```python
from build123d import *
from OCP.BRepFilletAPI import BRepFilletAPI_MakeChamfer

# Parameters (mm, degrees)
SKETCH2_W           = 18
SKETCH2_H           = 20
BOSS_EXTRUDE1_DEPTH = 22
SKETCH3_W           = 18
SKETCH3_H           = 20
BOSS_EXTRUDE2_DEPTH = 8
BOSS_EXTRUDE2_DRAFT = -25
SKETCH4_R           = 1.6
CUT_EXTRUDE1_DEPTH  = 18
CHAMFER1_SIZE       = 0.4
CHAMFER1_SIZE2      = 0.300994928


with BuildPart() as part:
    # Sketch2 → Boss-Extrude1 (new body)
    with BuildSketch(Plane.XY):
        Rectangle(SKETCH2_W, SKETCH2_H)
    extrude(amount=BOSS_EXTRUDE1_DEPTH)


with BuildPart() as boss_extrude2_tool:
    # Sketch3 → Boss-Extrude2 (with draft: the straight prism first)
    with BuildSketch(Plane(origin=(0, 0, 0), x_dir=(-1, 0, 0), z_dir=(0, 0, -1))):
        Rectangle(SKETCH3_W, SKETCH3_H)
    extrude(amount=BOSS_EXTRUDE2_DEPTH)
    # Boss-Extrude2: the draft: its side faces are tilted about the plane it starts from
    boss_extrude2_sides = [boss_extrude2_tool.faces().sort_by_distance(p)[0] for p in [
        (9, 0, -4),
        (0, -10, -4),
        (-9, 0, -4),
        (0, 10, -4),
    ]]
    draft(boss_extrude2_sides, Plane(origin=(0, 0, 0), x_dir=(-1, 0, 0), z_dir=(0, 0, -1)), BOSS_EXTRUDE2_DRAFT)


with BuildPart() as part_1:
    add(part.part)

    # Boss-Extrude2: add boss_extrude2_tool
    add(boss_extrude2_tool.part)

    # Sketch4 → Cut-Extrude1 (cut)
    with BuildSketch(Plane(origin=(9, 0, 0), x_dir=(0, 0, -1), z_dir=(1, 0, 0))):
        with Locations((-17, 5)):
            Circle(SKETCH4_R)
        with Locations((-9, 5)):
            Circle(SKETCH4_R)
        with Locations((-17, -5)):
            Circle(SKETCH4_R)
        with Locations((-9, -5)):
            Circle(SKETCH4_R)
    extrude(amount=-CUT_EXTRUDE1_DEPTH, mode=Mode.SUBTRACT)

    # Chamfer1: one chamfer whose edges measure the first distance from different faces: ONE call of the kernel's chamfer builder (chamfer() names one face for all edges)
    chamfer1_edges_1 = [part_1.edges().sort_by_distance(p)[0] for p in [
        (0, 13.730461265, -8),
    ]]
    chamfer1_side_1 = [part_1.faces().sort_by_distance(p)[0] for p in [
        (0, 11.971965146, -4.228892903),
    ]]
    chamfer1_edges_2 = [part_1.edges().sort_by_distance(p)[0] for p in [
        (12.730461265, 0, -8),
    ]]
    chamfer1_side_2 = [part_1.faces().sort_by_distance(p)[0] for p in [
        (10.962969576, 0, -4.20960184),
    ]]
    chamfer1_edges_3 = [part_1.edges().sort_by_distance(p)[0] for p in [
        (0, -13.730461265, -8),
    ]]
    chamfer1_side_3 = [part_1.faces().sort_by_distance(p)[0] for p in [
        (0, -11.971965146, -4.228892903),
    ]]
    chamfer1_edges_4 = [part_1.edges().sort_by_distance(p)[0] for p in [
        (-12.730461265, 0, -8),
    ]]
    chamfer1_side_4 = [part_1.faces().sort_by_distance(p)[0] for p in [
        (-10.962969576, 0, -4.20960184),
    ]]
    chamfer1 = BRepFilletAPI_MakeChamfer(part_1.part.solid().wrapped)
    for e in chamfer1_edges_1:
        chamfer1.Add(CHAMFER1_SIZE, CHAMFER1_SIZE2, e.wrapped, chamfer1_side_1[0].wrapped)  # the first distance lies on this face
    for e in chamfer1_edges_2:
        chamfer1.Add(CHAMFER1_SIZE, CHAMFER1_SIZE2, e.wrapped, chamfer1_side_2[0].wrapped)  # the first distance lies on this face
    for e in chamfer1_edges_3:
        chamfer1.Add(CHAMFER1_SIZE, CHAMFER1_SIZE2, e.wrapped, chamfer1_side_3[0].wrapped)  # the first distance lies on this face
    for e in chamfer1_edges_4:
        chamfer1.Add(CHAMFER1_SIZE, CHAMFER1_SIZE2, e.wrapped, chamfer1_side_4[0].wrapped)  # the first distance lies on this face
    add(Compound.cast(chamfer1.Shape()), mode=Mode.REPLACE)


solid = part_1.part
```
Check sheet for the modelled part. Datum: model origin and axes. Units: mm. A direction names the side the tool comes from. Give positions to 0.01 mm unless a question says otherwise; leave off trailing zeros. Order: outer loops, then holes, each group sorted by start corner. A loop starts at its lowest first (then second) coordinate and runs counter-clockwise, first axis right, second up. Notation, with made-up numbers: (73, 68.25) -> (98, 68.25) arc R20 cw to (98, 72.25) -> close; hole circle Ø9 at (14.5, 85.25). An arc over 180 degrees is marked (long way). Return JSON: item names as keys, results as strings.
1. Go/stop test with flat-tipped pins: P1, Ø5, axis at y = 5, z = 17, coming from the +X side; P2, Ø12, axis at x = -3, z = -1, coming from the +Y side; P3, Ø9, axis at x = 1, z = 8.5, coming from the -Y side; P4, Ø3, axis at y = -5, z = 9, coming from the +X side. Record where each tip stops, or that it passes through.
From the geometry:
{"P1": "x = 9", "P2": "y = 13.26", "P3": "y = -10", "P4": "through"}
2. Cross-section at D-D, the plane x = 9.5. Record the cut outline in (y, z).
From the geometry:
{"outline": "(-13.56, -7.64) -> (-13.43, -8) -> (13.43, -8) -> (13.56, -7.64) -> (10.5, -1.07) -> (-10.5, -1.07) -> close"}
3. Set-up check for faces 5 (the flat face through (0, 10, 11)), 6 (the flat face through (-9, 0, 11)), 7 (the flat face through (9, 0, 11)): record each of +Z, -Z, +X, -X, +Y, -Y from which the full face is reachable in a straight line by a thin tool's end or side.
From the geometry:
{"face 5": "+Z, +X, -X, +Y", "face 6": "+Z, -X, +Y, -Y", "face 7": "+Z, +X, +Y, -Y"}
4. Cross-section at C-C, the plane y = 5. Record the cut outline in (x, z).
From the geometry:
{"outline": "(-12.56, -7.64) -> (-12.43, -8) -> (12.43, -8) -> (12.56, -7.64) -> (9, 0) -> (9, 7.4) -> (-9, 7.4) -> (-9, 0) -> close; (-9, 10.6) -> (9, 10.6) -> (9, 15.4) -> (-9, 15.4) -> close; (-9, 18.6) -> (9, 18.6) -> (9, 22) -> (-9, 22) -> close"}
5. Mould release check, pull along Z, two halves, no side actions. Record for faces 1 (the flat face through (0, -10, 11)), 2 (the cylindrical face through (0.13, -4.93, 10.6)), 3 (the flat face through (0, 0, 22)), 4 (the cylindrical face through (0.13, 4.03, 10.27)): +Z half, -Z half, draft (parallel to the pull), parting line (faces both ways), or undercut.
From the geometry:
{"face 1": "draft", "face 2": "undercut", "face 3": "+Z half", "face 4": "undercut"}
6. Material ranges on probe 1 along Y at (x, z) = (1.5, 9); probe 2 along Z at (x, y) = (2.25, -4.5); probe 3 along X at (y, z) = (-5, 20.75), recorded low to high. Write a range as [from, to].
From the geometry:
{"probe 1": "[-10, -6.6], [-3.4, 3.4], [6.6, 10]", "probe 2": "[-8, 7.48], [10.52, 15.48], [18.52, 22]", "probe 3": "[-9, 9]"}
7. Cross-section at B-B, the plane z = 17. Record the cut outline in (x, y).
From the geometry:
{"outline": "(-9, -10) -> (9, -10) -> (9, -6.6) -> (-9, -6.6) -> close; (-9, -3.4) -> (9, -3.4) -> (9, 3.4) -> (-9, 3.4) -> close; (-9, 6.6) -> (9, 6.6) -> (9, 10) -> (-9, 10) -> close"}
8. Cross-section at A-A, the plane x = -2. Record the cut outline in (y, z), plus the area to 3 significant figures.
From the geometry:
{"outline": "(-13.56, -7.64) -> (-13.43, -8) -> (13.43, -8) -> (13.56, -7.64) -> (10, 0) -> (10, 22) -> (-10, 22) -> (-10, 0) -> close; hole circle Ø3.2 at (-5, 9); hole circle Ø3.2 at (-5, 17); hole circle Ø3.2 at (5, 9); hole circle Ø3.2 at (5, 17)", "area": "598 mm^2"}
